```python
from build123d import *

# Parameters (mm, degrees)
SKETCH_1_W          = 24.72
SKETCH_1_H          = 49.22
EXTRUDE_1_DEPTH     = 36
SKETCH_3_W          = 24.72
SKETCH_3_H          = 32
CUT_EXTRUDE_1_DEPTH = 46.22
SKETCH_4_R          = 1
SKETCH_4_R_2        = 10
SKETCH_4_W          = 20.72
SKETCH_4_H          = 20.22
CUT_EXTRUDE_2_DEPTH = 2
SKETCH_6_R          = 1
CUT_EXTRUDE_3_DEPTH = 6
SKETCH_7_R          = 10
EXTRUDE_2_DEPTH     = 3
SKETCH_8_R          = 1.25
CUT_EXTRUDE_4_DEPTH = 8
FILLET_1_R          = 2
FILLET_2_R          = 2
FILLET_3_SIZE       = 2
FILLET_4_R          = 2
FILLET_5_R          = 1
FILLET_6_R          = 1
FILLET_7_R          = 1
FILLET_8_R          = 1
FILLET_9_R          = 1
FILLET_10_R         = 1
SKETCH_9_R          = 3
CUT_EXTRUDE_5_DEPTH = 10


# Some blends are built 0.0001 mm under size
with BuildPart() as part:
    # 草图1 → 凸台-拉伸1 (new body)
    with BuildSketch(Plane.XY):
        with Locations((12.36, 24.61)):
            Rectangle(SKETCH_1_W, SKETCH_1_H)
    extrude(amount=EXTRUDE_1_DEPTH)

    # 草图3 → 切除-拉伸1 (cut)
    with BuildSketch(Plane.XZ):
        with Locations((12.36, 18)):
            Rectangle(SKETCH_3_W, SKETCH_3_H)
    extrude(amount=-CUT_EXTRUDE_1_DEPTH, mode=Mode.SUBTRACT)

    # 草图4 → 切除-拉伸2 (cut)
    with BuildSketch(Plane.XY.offset(2)):
        with Locations((2, 2.36)):
            Circle(SKETCH_4_R)
        with Locations((22.72, 2.36)):
            Circle(SKETCH_4_R)
        with Locations((22.72, 26.81)):
            Circle(SKETCH_4_R)
        with Locations((2, 26.81)):
            Circle(SKETCH_4_R)
        with Locations((12.36, 36.11)):
            Circle(SKETCH_4_R_2)
        with Locations((12.36, 14.11)):
            Rectangle(SKETCH_4_W, SKETCH_4_H)
    extrude(amount=-CUT_EXTRUDE_2_DEPTH, mode=Mode.SUBTRACT)

    # 草图6 → 切除-拉伸3 (cut)
    with BuildSketch(Plane.XY.offset(36)):
        with BuildLine():
            Line((5.4, 27.996527822), (5.4, 28))
            Line((5.4, 28), (19.4, 28))
            Line((19.4, 28), (19.4, 27.940836898))
            ThreePointArc((19.4, 27.940836898), (21.640245754, 31.218722824), (22.428407613, 35.11))
            ThreePointArc((22.428407613, 35.11), (8.573804918, 44.337244337), (5.4, 27.996527822))
        make_face()
        with BuildLine():
            Line((19.4, 28), (5.4, 28))
            Line((5.4, 28), (5.4, 27.996527822))
            ThreePointArc((5.4, 27.996527822), (12.388628696, 25.110079118), (19.4, 27.940836898))
            Line((19.4, 27.940836898), (19.4, 28))
        make_face()
        with BuildLine():
            ThreePointArc((19.4, 27.940836898), (12.388628696, 25.110079118), (5.4, 27.996527822))
            Line((5.4, 27.996527822), (5.4, 0))
            Line((5.4, 0), (19.4, 0))
            Line((19.4, 0), (19.4, 27.940836898))
        make_face()
        with Locations((2, 26.81)):
            Circle(SKETCH_6_R)
        with Locations((22.72, 6.11)):
            Circle(SKETCH_6_R)
        with Locations((2, 6.11)):
            Circle(SKETCH_6_R)
        with Locations((22.72, 26.81)):
            Circle(SKETCH_6_R)
    extrude(amount=-CUT_EXTRUDE_3_DEPTH, mode=Mode.SUBTRACT)

    # 草图7 → 凸台-拉伸2 (add)
    with BuildSketch(Plane(origin=(0, 49.22, 0), x_dir=(1, 0, 0), z_dir=(0, 1, 0))):
        with Locations(Location((12.36, -20, 0), (0, 0, 270))):
            Circle(SKETCH_7_R)
    extrude(amount=EXTRUDE_2_DEPTH)

    # 草图8 → 切除-拉伸4 (cut)
    with BuildSketch(Plane(origin=(0, 52.22, 0), x_dir=(1, 0, 0), z_dir=(0, 1, 0))):
        with Locations(Location((12.36, -13, 0), (0, 0, 270))):
            Circle(SKETCH_8_R)
        with Locations(Location((12.36, -27, 0), (0, 0, 270))):
            Circle(SKETCH_8_R)
        with Locations(Location((19.36, -20, 0), (0, 0, 270))):
            Circle(SKETCH_8_R)
        with Locations(Location((5.36, -20, 0), (0, 0, 270))):
            Circle(SKETCH_8_R)
    extrude(amount=-CUT_EXTRUDE_4_DEPTH, mode=Mode.SUBTRACT)

    # 圆角1
    fillet_1_edges = [part.edges().sort_by_distance(p)[0] for p in [
        (12.36, 46.22, 11.75),
    ]]
    fillet(fillet_1_edges, radius=FILLET_1_R)

    # 圆角2
    fillet_2_edges = [part.edges().sort_by_distance(p)[0] for p in [
        (19.36, 46.22, 18.75),
    ]]
    fillet(fillet_2_edges, radius=FILLET_2_R)

    # 圆角3
    # a fillet whose section is not a circle: 2 mm, written as the material it takes off along each edge
    with BuildSketch(Plane(origin=(12.36, 46.22, 27), x_dir=(0, 0, 1), z_dir=(-1, 0, 0))) as fillet_3_piece_1:
        with BuildLine():
            Bezier((1.25 + FILLET_3_SIZE, 0), (1.25, 0), (1.25, FILLET_3_SIZE), weights=[1, 1, 1])
            Line((1.25, FILLET_3_SIZE), (1.25, 0))
            Line((1.25, 0), (1.25 + FILLET_3_SIZE, 0))
        make_face()
    revolve(axis=Axis((12.36, 46.22, 27), (0, 1, 0)), mode=Mode.SUBTRACT)

    # 圆角4
    fillet_4_edges = [part.edges().sort_by_distance(p)[0] for p in [
        (5.36, 46.22, 18.75),
    ]]
    fillet(fillet_4_edges, radius=FILLET_4_R)

    # 圆角5
    fillet_5_edges = [part.edges().sort_by_distance(p)[0] for p in [
        (0, 24.61, 36),
    ]]
    fillet(fillet_5_edges, radius=FILLET_5_R - 0.0001)  # a hair under: the kernel refuses the full size

    # 圆角6
    fillet_6_edges = [part.edges().sort_by_distance(p)[0] for p in [
        (24.72, 24.61, 36),
    ]]
    fillet(fillet_6_edges, radius=FILLET_6_R - 0.0001)  # a hair under: the kernel refuses the full size

    # 圆角7
    fillet_7_edges = [part.edges().sort_by_distance(p)[0] for p in [
        (0, 24.61, 0),
    ]]
    fillet(fillet_7_edges, radius=FILLET_7_R - 0.0001)  # a hair under: the kernel refuses the full size

    # 圆角8
    fillet_8_edges = [part.edges().sort_by_distance(p)[0] for p in [
        (24.72, 24.61, 0),
    ]]
    fillet(fillet_8_edges, radius=FILLET_8_R - 0.0001)  # a hair under: the kernel refuses the full size

    # 圆角9
    fillet_9_edges = [part.edges().sort_by_distance(p)[0] for p in [
        (19.4, 13.970418449, 34),
    ]]
    fillet(fillet_9_edges, radius=FILLET_9_R)

    # 圆角10
    fillet_10_edges = [part.edges().sort_by_distance(p)[0] for p in [
        (5.4, 13.998263911, 34),
    ]]
    fillet(fillet_10_edges, radius=FILLET_10_R)

    # 草图9 → 切除-拉伸5 (cut)
    with BuildSketch(Plane(origin=(0, 52.22, 0), x_dir=(1, 0, 0), z_dir=(0, 1, 0))):
        with Locations(Location((12.36, -20, 0), (0, 0, 270))):
            Circle(SKETCH_9_R)
    extrude(amount=-CUT_EXTRUDE_5_DEPTH, mode=Mode.SUBTRACT)


solid = part.part
```
Can you work these out from the model? Positions are in its coordinate system, mm. A direction names the side the tool comes from. Give positions to 0.01 mm unless a question says otherwise; leave off trailing zeros. Write each loop counter-clockwise with the first axis right and the second up, starting at its lowest first coordinate (ties: lowest second). Pieces come first, ordered by that corner, then holes. Notation, with made-up numbers: (25.25, -7) - (58.25, -7) arc R18 cw to (58.25, 27) - close; hole circle Ø10 at (12.5, 51.25). An arc over 180 degrees is marked (long way). Write item = value, one per line. Start each with the question number.
1. Please list where these lines run through material, in increasing order: line 1 (Y direction, x = 22.72, z = 35.2); line 2 (Y direction, x = 8, z = 12); line 3 (Z direction, x = 12, y = 46).
2. For pin 1 (1.6 mm diameter, centred on x = 10, z = 0.5, fed in from +Y); pin 2 (3 mm diameter, centred on x = 12.36, z = 13, fed in from -Y); pin 3 (1.2 mm diameter, centred on x = 2, y = 6.11, fed in from +Z), each with a flat end and sliding along its axis, tell me the tip position at first contact or that it passes through.
3. Imagine slicing it at A-A (z = 20). Please give me the cut outline in (x, y).
4. On a 3-axis mill with a long thin cutter (end or side, diameter ignored), from which of +Z, -Z, +X, -X, +Y, -Y can I reach the whole of each face in a straight line? I mean faces 1 (the face through (1, 2.4, 1)), 2 (the face through (1.87, 7.1, 35.01)), 3 (the face through (9, 46.22, 18)), 4 (the face through (12.2, 49.22, 9.7)), 5 (the face through (11.881, 50.248, 28.155)). Say none if no direction works.
5. Thinking about a two-plate mould opening in X: for faces 6 (the face through (12, 0, 1)), 7 (the face through (12, 24.22, 1)), 8 (the face through (15.36, 50.7, 29.54)), 9 (the face through (2, 14, 1)), which applies, released by +X, released by -X, zero draft, split by the parting line, or undercut?
6. Imagine slicing it at C-C (z = 13). Please give me the cut outline in (x, y).
7. Imagine slicing it at B-B (y = 11). Please give me the cut outline in (x, z).
8. Imagine slicing it at D-D (y = 31). Please give me the cut outline in (x, z).
Worked answers:
q1.line_1 = 0 to 5.11, 7.11 to 25.81, 27.81 to 49.22
q1.line_2 = 46.22 to 52.22
q1.line_3 = 34 to 36
q2.pin_1 = 49.22
q2.pin_2 = 47.25
q2.pin_3 = 2
q3.outline = (0, 46.22) - (2.11, 46.22) arc R2 ccw to (4.11, 48.22) - (4.11, 52.22) - (2.36, 52.22) - (2.36, 49.22) - (0, 49.22) - close; (6.61, 48.22) arc R2 ccw to (8.61, 46.22) - (9.36, 46.22) - (9.36, 52.22) - (6.61, 52.22) - close; (15.36, 46.22) - (16.11, 46.22) arc R2 ccw to (18.11, 48.22) - (18.11, 52.22) - (15.36, 52.22) - close; (20.61, 48.22) arc R2 ccw to (22.61, 46.22) - (24.72, 46.22) - (24.72, 49.22) - (22.36, 49.22) - (22.36, 52.22) - (20.61, 52.22) - close
q4.face_1 = -Z
q4.face_2 = +Z
q4.face_3 = +X, -X, -Y
q4.face_4 = +Y
q4.face_5 = +Y, -Y
q5.face_6 = zero draft
q5.face_7 = undercut
q5.face_8 = split by the parting line
q5.face_9 = undercut
q6.outline = (0, 46.22) - (9.11, 46.22) arc R2 ccw to (11.11, 48.22) - (11.11, 52.22) - (5.22, 52.22) - (5.22, 49.22) - (0, 49.22) - close; (13.61, 48.22) arc R2 ccw to (15.61, 46.22) - (24.72, 46.22) - (24.72, 49.22) - (19.5, 49.22) - (19.5, 52.22) - (13.61, 52.22) - close
q7.outline = (0, 1) arc R1 ccw to (1, 0) - (2, 0) - (2, 2) - (0, 2) - close; (0, 34) - (4.4, 34) arc R1 ccw to (5.4, 35) - (5.4, 36) - (1, 36) arc R1 ccw to (0, 35) - close; (19.4, 35) arc R1 ccw to (20.4, 34) - (24.72, 34) - (24.72, 35) arc R1 ccw to (23.72, 36) - (19.4, 36) - close; (22.72, 0) - (23.72, 0) arc R1 ccw to (24.72, 1) - (24.72, 2) - (22.72, 2) - close
q8.outline = (0, 1) arc R1 ccw to (1, 0) - (3.76, 0) - (3.76, 2) - (0, 2) - close; (0, 34) - (3.31, 34) - (3.31, 36) - (1, 36) arc R1 ccw to (0, 35) - close; (20.96, 0) - (23.72, 0) arc R1 ccw to (24.72, 1) - (24.72, 2) - (20.96, 2) - close; (21.54, 34) - (24.72, 34) - (24.72, 35) arc R1 ccw to (23.72, 36) - (21.54, 36) - close
